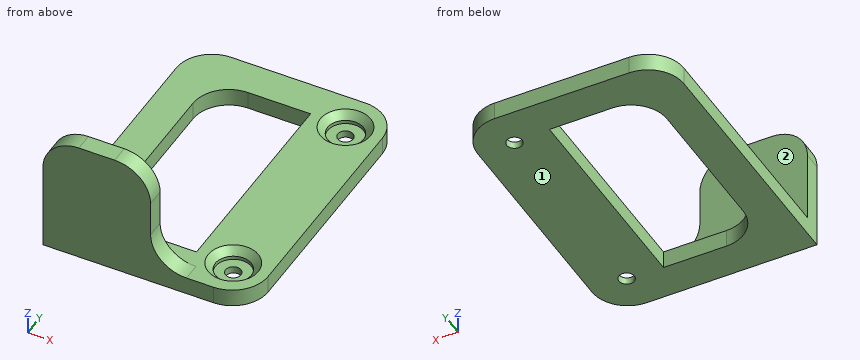
Autodesk Inventor part; units mm, degrees
ref_plane "YZ Plane" through (0, 0, 0) normal (1, 0, 0) x (0, 1, 0)
ref_plane "XZ Plane" through (0, 0, 0) normal (0, 1, 0) x (-1, 0, 0)
ref_plane "XY Plane" through (0, 0, 0) normal (0, 0, 1) x (1, 0, 0)
ref_plane "Work Plane1" through (0, 0, 0) normal (0, 0, 1) x (1, 0, 0)
sketch "Sketch1" plane through (0, 0, 0) normal (0, 0, 1) x (1, 0, 0)
  circle A0 centre (-80, 29.5) radius 2.15
  circle A1 centre (-80, -29.5) radius 2.15
  line L0 (-127.5, 40) -> (-70, 40)
  line L1 (-70, 40) -> (-70, -40)
  line L2 (-70, -40) -> (-127.5, -40)
  line L3 (-127.5, -40) -> (-127.5, 40)
  line L4 (87.5, 40) -> (-87.5, 40)
  line L5 (-87.5, -40) -> (87.5, -40)
  line L6 (-97.5, 30) -> (-97.5, -30)
  line L7 (-117.5, 30) -> (-90, 30)
  line L8 (-90, 30) -> (-90, -30)
  line L9 (-90, -30) -> (-117.5, -30)
  line L10 (-117.5, -30) -> (-117.5, 30)
  point P0 (0, 0)
  point P1 (-117.5, 0)
  point P2 (-127.5, 0)
  dimension "d0" = 10
  dimension "d1" = 30
  dimension "d2" = 10
  dimension "d3" = 10
  dimension "d4" = 10
extrude "Extrusion1" add sketch "Sketch1" along normal blind 5
sketch "Sketch2" plane through (0, 0, 5) normal (0, 0, 1) x (1, 0, 0)
  line L0 (-127.5, -40) -> (-70, -40)
  line L1 (-127.5, -40) -> (-97.5, -40)
  line L2 (-97.5, -40) -> (-97.5, -35)
  line L3 (-97.5, -35) -> (-127.5, -35)
  line L4 (-127.5, -35) -> (-127.5, -40)
  line L5 (-97.5, 30) -> (-97.5, -30)
  point P0 (0, 0)
  dimension "d7" = 5
  dimension "d8" = 30
extrude "Extrusion2" add sketch "Sketch2" along normal blind 30
sketch "Sketch3" plane through (0, 0, 5) normal (0, 0, 1) x (1, 0, 0)
  circle A0 centre (-80, 29.5) radius 2.15
  circle A1 centre (-80, 29.5) radius 5
  circle A2 centre (-80, -29.5) radius 2.15
  circle A3 centre (-80, -29.5) radius 5
  point P0 (0, 0)
  dimension "d11" = 10
  dimension "d12" = 10
extrude "Extrusion3" cut sketch "Sketch3" against normal blind 3
chamfer "Chamfer1" distance 2 angle 45 2 edges at (-85, 29.5, 5) (-85, -29.5, 5)
fillet "Fillet1" radius 10 3 edges at (-127.5, -37.5, 35) (-97.5, -37.5, 35) (-97.5, -37.5, 5)
fillet "Fillet2" radius 10 5 edges at (-127.5, 40, 2.5) (-117.5, 30, 2.5) (-117.5, -30, 2.5) (-70, 40, 2.5) (-70, -40, 2.5)
properties part number "led 7 seg v3_stand"
Verification items for the finished model (mm, model axes). Face numbers are marked on the shaded views. A direction names the side the tool comes from. Round coordinates to 2 decimals unless told otherwise and drop trailing zeros. Write each loop counter-clockwise with the first axis right and the second up, starting at its lowest first coordinate (ties: lowest second). Pieces come first, ordered by that corner, then holes.
1. Scan lines: L1, parallel to Y at x = -80, z = 0.4; L2, parallel to Y at x = -80, z = 2.45; L3, parallel to Z at x = -123.5, y = -20. Record each from-to range of solid material in increasing order.
2. Gauge pin test, flat ends, axial feed: P1, Ø2.5, axis at x = -80, y = 29.5, coming from the +Z side; P2, Ø10, axis at x = -109, z = 28, coming from the +Y side; P3, Ø7, axis at x = -80, y = -29.5, coming from the +Z side; P4, Ø4, axis at x = -90.5, y = 26.5, coming from the +Z side. Record the tip position at first contact, or that the pin passes through.
3. Section check B-B on x = -115. Enter the section's corners in (y, z).
4. Access from +Z, -Z, +X, -X, +Y, -Y to the whole of each face (thin tool, end or side, straight path). Record for the marked faces 1 and 2.
5. Section check A-A on y = -12. Enter the section's corners in (x, z), plus the area to 3 significant figures.
6. Section check C-C on z = 16. Enter the section's corners in (x, y), plus the area to 3 significant figures.
7. Section check D-D on x = -92. Enter the section's corners in (y, z), plus the area to 3 significant figures.
Answer:
1. L1: y = -40 to -31.65, -27.35 to 27.35, 31.65 to 40
1. L2: y = -40 to -34.5, -24.5 to 24.5, 34.5 to 40
1. L3: z = 0 to 5
2. P1: passes through
2. P2: stops at y = -35
2. P3: stops at z = 2
2. P4: stops at z = 5
3. outline: (-40, 0) - (-26.61, 0) - (-26.61, 5) - (-35, 5) - (-35, 35) - (-40, 35) - close; (26.61, 0) - (40, 0) - (40, 5) - (26.61, 5) - close
4. face 1: -Z, +X, -X, +Y, -Y
4. face 2: +Z, +X, -X, +Y
5. outline: (-127.5, 0) - (-117.5, 0) - (-117.5, 5) - (-127.5, 5) - close; (-90, 0) - (-70, 0) - (-70, 5) - (-90, 5) - close
5. area: 150 mm2
6. outline: (-127.5, -40) - (-97.5, -40) - (-97.5, -35) - (-127.5, -35) - close
6. area: 150 mm2
7. outline: (-40, 0) - (-30, 0) - (-30, 5) - (-35, 5) - (-35, 6.07) - (-40, 6.07) - close; (30, 0) - (40, 0) - (40, 5) - (30, 5) - close
7. area: 105 mm2
